Design review of the part built by this model. Coordinates are the model's own, in mm. A direction names the side the tool comes from. Coordinates: 2 decimals unless noted, no trailing zeros. Write each loop counter-clockwise with the first axis right and the second up, starting at its lowest first coordinate (ties: lowest second). Pieces come first, ordered by that corner, then holes. Notation, with made-up numbers: (46.25, 72) - (90.25, 72) arc R22 cw to (90.25, 99) - close; hole circle Ø11 at (77, 39). An arc over 180 degrees is marked (long way). Answer as a JSON object with one key per item and string values.
```python
from build123d import *

# Parameters (mm, degrees)
F0_W     = 65
F0_H     = 65
F5_DEPTH = 58
F1_R     = 25.5
F6_DEPTH = 25
F3_R     = 4.2
F7_DEPTH = 134
F4_R     = 7.6
F8_DEPTH = 47
F2_R     = 19.5
F9_DEPTH = 33


with BuildPart() as f5:
    # F0 (on Top) → F5 (new body)
    with BuildSketch(Plane.XY):
        Rectangle(F0_W, F0_H)
    extrude(amount=F5_DEPTH)

    # F1 (on face) → F6 (join)
    with BuildSketch(Plane.XY):
        Circle(F1_R)
    extrude(amount=F6_DEPTH)

    # F3 (on Top) → F7 (cut)
    with BuildSketch(Plane.XY):
        Circle(F3_R)
    extrude(amount=F7_DEPTH, mode=Mode.SUBTRACT)

    # F4 (on Top) → F8 (cut)
    with BuildSketch(Plane.XY):
        Circle(F4_R)
    extrude(amount=F8_DEPTH, mode=Mode.SUBTRACT)

    # F2 (on Top) → F9 (cut)
    with BuildSketch(Plane.XY):
        Circle(F2_R)
    extrude(amount=F9_DEPTH, mode=Mode.SUBTRACT)


solid = f5.part
```
(1) The part is to be moulded in two halves that separate along X. For faces 3 (the face through (-32.5, 0, 29)), 4 (the face through (-2.539, 19.334, 16.269)), 5 (the face through (0, 32.5, 29)), say which applies: pulls with the +X half, pulls with the -X half, needs draft (parallel to the pull), parting line crosses it, or undercut.
Solved:
{"face 3": "pulls with the -X half", "face 4": "undercut", "face 5": "needs draft"}
(2) Take a section at A-A, the plane x = 0. Write out the cut boundary in (y, z), and give its area (3 significant figures).
Solved:
{"outline": "(-32.5, 0) - (-19.5, 0) - (-19.5, 33) - (-7.6, 33) - (-7.6, 47) - (-4.2, 47) - (-4.2, 58) - (-32.5, 58) - close; (4.2, 47) - (7.6, 47) - (7.6, 33) - (19.5, 33) - (19.5, 0) - (32.5, 0) - (32.5, 58) - (4.2, 58) - close", "area": "2,180 mm^2"}
(3) Tool access review of faces 1 (the face through (3.3, -3.3, 47)), 2 (the face through (4.006, 1.262, 52.423)): name each direction out of +Z, -Z, +X, -X, +Y, -Y from which nothing blocks a thin tool from reaching the whole face with its end or side.
Solved:
{"face 1": "-Z", "face 2": "+Z, -Z"}
(4) To check wall thickness, follow line 1 (X direction, y = 0, z = 50.75); line 2 (Y direction, x = 0, z = 26); line 3 (X direction, y = 0, z = 37.75). State the ranges of each line that lie inside material, in increasing order. Write a range as from..to.
Solved:
{"line 1": "x = -32.5..-4.2, 4.2..32.5", "line 2": "y = -32.5..-19.5, 19.5..32.5", "line 3": "x = -32.5..-7.6, 7.6..32.5"}
(5) For pin 1 (8 mm diameter, centred on x = 11.5, y = 11.5, fed in from -Z); pin 2 (7.5 mm diameter, centred on x = -3.5, y = -3.5, fed in from -Z), all flat-tipped, find the tip position at first contact; note any pin that passes through.
Solved:
{"pin 1": "stops at z = 0", "pin 2": "stops at z = 33"}
(6) Take a section at D-D, the plane z = 44. Write out the cut boundary in (x, y).
Solved:
{"outline": "(-32.5, -32.5) - (32.5, -32.5) - (32.5, 32.5) - (-32.5, 32.5) - close; hole circle Ø15.2 at (0, 0)"}
(7) Take a section at C-C, the plane z = 28. Write out the cut boundary in (x, y).
Solved:
{"outline": "(-32.5, -32.5) - (32.5, -32.5) - (32.5, 32.5) - (-32.5, 32.5) - close; hole circle Ø39 at (0, 0)"}
